Autodesk Inventor part; units mm, degrees
ref_plane "YZ Plane" through (0, 0, 0) normal (1, 0, 0) x (0, 1, 0)
ref_plane "XZ Plane" through (0, 0, 0) normal (0, 1, 0) x (-1, 0, 0)
ref_plane "XY Plane" through (0, 0, 0) normal (0, 0, 1) x (1, 0, 0)
sketch "Skizze1" plane through (0, 0, 0) normal (0, 0, 1) x (1, 0, 0)
  line L0 (0, 0) -> (35, 0)
  line L1 (35, 0) -> (35, 22)
  line L2 (35, 22) -> (0, 22)
  line L3 (0, 22) -> (0, 0)
  dimension "d0" = 35
  dimension "d1" = 22
extrude "Extrusion1" add sketch "Skizze1" along normal blind 1.5
sketch "Skizze2" plane through (0, 0, 1.5) normal (0, 0, 1) x (1, 0, 0)
  line L0 (0, 0) -> (35, 0) construction
  line L1 (35, 0) -> (35, 22) construction
  line L2 (35, 22) -> (0, 22) construction
  line L3 (0, 22) -> (0, 0) construction
  line L4 (35, 0) -> (35, 22) construction
  line L5 (35, 11) -> (0, 11) construction
  line L6 (0, 22) -> (0, 0) construction
  line L7 (0, 0) -> (35, 0) construction
  line L8 (17.5, 0) -> (17.5, 22) construction
  line L9 (35, 22) -> (0, 22) construction
  point P0 (32.5, 19.5)
  point P1 (32.5, 2.5)
  point P2 (2.5, 19.5)
  point P3 (2.5, 2.5)
  dimension "d4" = 2.5
  dimension "d5" = 2.5
hole "Bohrung1" at (32.5, 19.5, 1.5) at (32.5, 2.5, 1.5) at (2.5, 2.5, 1.5) at (2.5, 19.5, 1.5) direction (0, 0, -1) diameter 3 end through all
sketch "Skizze3" plane through (0, 0, 1.5) normal (0, 0, 1) x (1, 0, 0)
  line L0 (35, 0) -> (35, 22) construction
  circle A0 centre (32.5, 2.5) radius 1.5 construction
  line L1 (32.5, 9.73) -> (32.5, 12.27) construction
  point P0 (0, 0)
  point P1 (32.5, 7.19)
  point P2 (32.5, 14.81)
  point P3 (32.5, 11)
  point P4 (35, 11)
  dimension "d15" = 2.54
hole "Bohrung2" at (32.5, 7.19, 1.5) at (32.5, 9.73, 1.5) at (32.5, 12.27, 1.5) at (32.5, 14.81, 1.5) direction (0, 0, -1) diameter 0.8 end through all
sketch "Skizze4" plane through (0, 0, 0) normal (0, 0, -1) x (-1, 0, 0)
  line L0 (0, 22) -> (0, 0) construction
  line L1 (0, 11) -> (-35, 11) construction
  line L2 (-35, 0) -> (-35, 22) construction
  line L3 (-10.1588, 15.75) -> (-10.1588, 6.25) construction
  point P0 (-6.8, 14.3588)
  point P1 (-13.5175, 14.3588)
  point P2 (-6.8, 7.6412)
  point P3 (-13.5175, 7.6412)
  dimension "d27" = 6.7175
  dimension "d29" = 6.7175
  dimension "d30" = 3.6355
  dimension "d31" = 6.8
hole "Bohrung3" at (6.8, 14.3588, 0) at (10.1588, 15.75, 0) at (13.5175, 14.3588, 0) at (6.8, 7.6412, 0) at (10.1588, 6.25, 0) at (13.5175, 7.6412, 0) direction (0, 0, 1) diameter 0.8 end through all
sketch "Skizze5" plane through (0, 0, 0) normal (0, 0, -1) x (-1, 0, 0)
  line L0 (-35, 0) -> (-35, 22) construction
  line L1 (-35, 11) -> (0, 11) construction
  line L2 (0, 22) -> (0, 0) construction
  point P0 (-22.26, 8.46)
  point P1 (-24.8, 11)
  point P2 (-22.26, 13.54)
  dimension "d39" = 5.08
  dimension "d40" = 2.54
  dimension "d41" = 10.2
hole "Bohrung4" at (22.26, 8.46, 0) at (24.8, 11, 0) at (22.26, 13.54, 0) direction (0, 0, 1) diameter 0.8 end through all
properties part number "Platine" material "LCP-Kunststoff"
Source: CAD feature listing. Evaluate the final solid. Frame: model axes, mm. Give positions to 0.01 mm unless a question says otherwise; leave off trailing zeros. Write each loop counter-clockwise with the first axis right and the second up, starting at its lowest first coordinate (ties: lowest second). Pieces come first, ordered by that corner, then holes.
1. Material intervals for line 1 along Y through (x, z) = (22.26, 0.4); line 2 along X through (y, z) = (13.54, 0.5); line 3 along X through (y, z) = (7.19, 0.65), sorted ascending.
2. Pull-direction query (X, two-part tool) for faces 1 (the face through (17, 11, 1.5)), 2 (the face through (13.397, 8.023, 0.76)), 3 (the face through (0, 11, 1)); classes: +X half, -X half, draft (parallel to the pull), parting line (faces both ways), or undercut.
3. Section query A-A (x = 6.8). Return the cut outline in (y, z).
4. Section query D-D (x = 32.5). Return the cut outline in (y, z).
5. Section query C-C (y = 11). Return the cut outline in (x, z), then the cut area to 3 significant figures.
6. Section query B-B (y = 2.5). Return the cut outline in (x, z), then the cut area to 3 significant figures.
Output values:
1. line 1: y = 0 to 8.06, 8.86 to 13.14, 13.94 to 22
1. line 2: x = 0 to 21.86, 22.66 to 35
1. line 3: x = 0 to 32.1, 32.9 to 35
2. face 1: draft
2. face 2: undercut
2. face 3: -X half
3. outline: (0, 0) - (7.24, 0) - (7.24, 1.5) - (0, 1.5) - close; (8.04, 0) - (13.96, 0) - (13.96, 1.5) - (8.04, 1.5) - close; (14.76, 0) - (22, 0) - (22, 1.5) - (14.76, 1.5) - close
4. outline: (0, 0) - (1, 0) - (1, 1.5) - (0, 1.5) - close; (4, 0) - (6.79, 0) - (6.79, 1.5) - (4, 1.5) - close; (7.59, 0) - (9.33, 0) - (9.33, 1.5) - (7.59, 1.5) - close; (10.13, 0) - (11.87, 0) - (11.87, 1.5) - (10.13, 1.5) - close; (12.67, 0) - (14.41, 0) - (14.41, 1.5) - (12.67, 1.5) - close; (15.21, 0) - (18, 0) - (18, 1.5) - (15.21, 1.5) - close; (21, 0) - (22, 0) - (22, 1.5) - (21, 1.5) - close
5. outline: (0, 0) - (24.4, 0) - (24.4, 1.5) - (0, 1.5) - close; (25.2, 0) - (35, 0) - (35, 1.5) - (25.2, 1.5) - close
5. area: 51.3 mm2
6. outline: (0, 0) - (1, 0) - (1, 1.5) - (0, 1.5) - close; (4, 0) - (31, 0) - (31, 1.5) - (4, 1.5) - close; (34, 0) - (35, 0) - (35, 1.5) - (34, 1.5) - close
6. area: 43.5 mm2
